Input: part model. Units: mm. Frame: model coordinates. Face numbers are marked on the shaded views. A direction names the side the tool comes from. Round coordinates to 2 decimals unless told otherwise and drop trailing zeros. Write each loop counter-clockwise with the first axis right and the second up, starting at its lowest first coordinate (ties: lowest second). Pieces come first, ordered by that corner, then holes. Notation, with made-up numbers: (-31.5, 41.5) -> (-11.5, 41.5) arc R13 cw to (-11.5, 56.5) -> close; hole circle Ø8 at (-17.5, 25.5). An arc over 180 degrees is marked (long way). Write item = value, one per line. Start each with the question number.
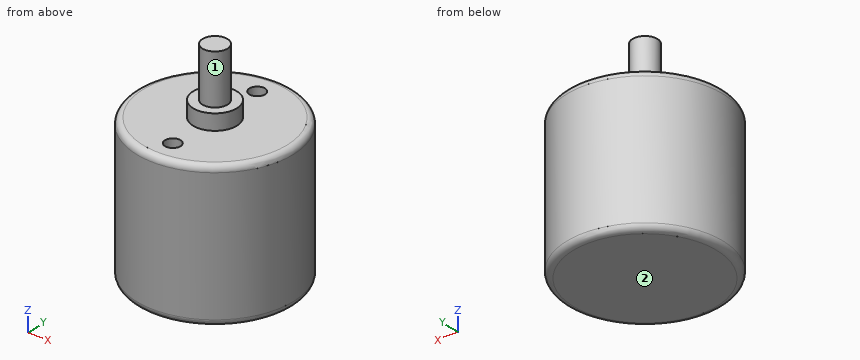
```python
from build123d import *

# Parameters (mm, degrees)
ESBO_O1_R                = 12.5
RESSALTO_EXTRUS_O1_DEPTH = 23
ESBO_O2_R                = 3.5
RESSALTO_EXTRUS_O2_DEPTH = 2.5
FILETE1_R                = 1
ESBO_O3_R                = 2
RESSALTO_EXTRUS_O3_DEPTH = 8
ESBO_O4_R                = 1.25
CORTE_EXTRUS_O1_DEPTH    = 10


with BuildPart() as part:
    # Esboço1 → Ressalto-extrusão1 (new body)
    with BuildSketch(Plane.XY):
        Circle(ESBO_O1_R)
    extrude(amount=RESSALTO_EXTRUS_O1_DEPTH)

    # Esboço2 → Ressalto-extrusão2 (add)
    with BuildSketch(Plane.XY.offset(23)):
        Circle(ESBO_O2_R)
    extrude(amount=RESSALTO_EXTRUS_O2_DEPTH)

    # Filete1
    filete1_edges = [part.edges().sort_by_distance(p)[0] for p in [
        (-12.5, 0, 0),
        (-12.5, 0, 23),
    ]]
    fillet(filete1_edges, radius=FILETE1_R)

    # Esboço3 → Ressalto-extrusão3 (add)
    with BuildSketch(Plane.XY.offset(25.5)):
        Circle(ESBO_O3_R)
    extrude(amount=RESSALTO_EXTRUS_O3_DEPTH)

    # Esboço4 → Corte-extrusão1 (cut)
    with BuildSketch(Plane.XY.offset(23)):
        with Locations((0, 8.5)):
            Circle(ESBO_O4_R)
        with Locations((0, -8.5)):
            Circle(ESBO_O4_R)
    extrude(amount=-CORTE_EXTRUS_O1_DEPTH, mode=Mode.SUBTRACT)


solid = part.part
```
1. Section B-B (z = 21). Output: boundary loops of the cut face in (x, y).
2. Line query: line 1 along Y through (x, z) = (0, 19); line 2 along Z through (x, y) = (6.5, 0.25); line 3 along Y through (x, z) = (0, 22.5). Output: solid intervals per line, ascending.
3. Pin query (flat end, axial travel): P1, Ø5, axis at x = -8.5, y = 4, coming from the +Z side; P2, Ø8, axis at x = -3.5, z = 26, coming from the +Y side; P3, Ø4, axis at x = 0.5, y = 10, coming from the -Z side; P4, Ø8, axis at x = 4, z = 28, coming from the -Y side. Return the tip coordinate at first contact, or that it passes through.
4. Reachability of the marked faces 1 and 2 from +Z, -Z, +X, -X, +Y, -Y: full face, straight path, thin tool, end or side. Return the list, or none.
5. Section A-A (y = 0). Output: boundary loops of the cut face in (x, z), then the cut area to 3 significant figures.
Check sheet entries:
q1.outline = circle Ø25 at (0, 0); hole circle Ø2.5 at (0, -8.5); hole circle Ø2.5 at (0, 8.5)
q2.line_1 = -12.5 to -9.75, -7.25 to 7.25, 9.75 to 12.5
q2.line_2 = 0 to 23
q2.line_3 = -12.37 to -9.75, -7.25 to 7.25, 9.75 to 12.37
q3.P1 = 23
q3.P2 = 12.3
q3.P3 = 0
q3.P4 = -3.39
q4.face_1 = +Z
q4.face_2 = -Z, +X, -X, +Y, -Y
q5.outline = (-12.5, 1) arc R1 ccw to (-11.5, 0) -> (11.5, 0) arc R1 ccw to (12.5, 1) -> (12.5, 22) arc R1 ccw to (11.5, 23) -> (3.5, 23) -> (3.5, 25.5) -> (2, 25.5) -> (2, 33.5) -> (-2, 33.5) -> (-2, 25.5) -> (-3.5, 25.5) -> (-3.5, 23) -> (-11.5, 23) arc R1 ccw to (-12.5, 22) -> close
q5.area = 624 mm2
